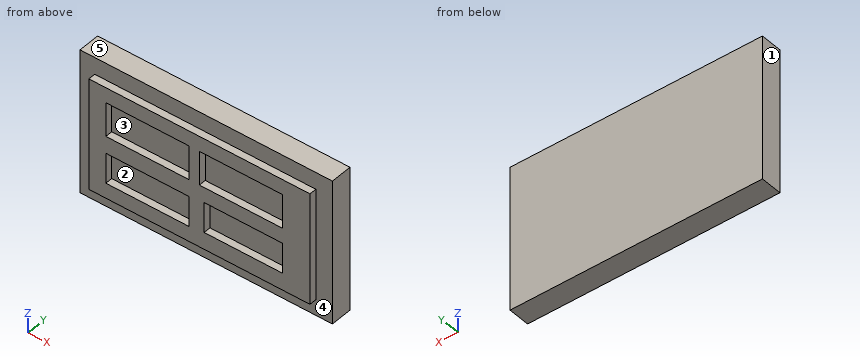
from build123d import *

# Parameters (mm, degrees)
F0_W        = 30.6613992434
F0_H        = 15.4617307708
F0_W_2      = 11.5307830274
F0_H_2      = 4.1930116713
F0_W_3      = 10.8756236732
F0_H_3      = 4.7171385959
F0_W_4      = 11.5307817468
F1_DEPTH    = 1
F0_W_5      = 35
F0_H_4      = 20
F2_DEPTH    = 2
F1_FACE_W   = 30.6613992434
F1_FACE_H   = 15.4617307708
F1_FACE_W_2 = 11.5307830274
F1_FACE_H_2 = 4.1930116713
F1_FACE_W_3 = 10.8756236732
F1_FACE_H_3 = 4.7171385959
F1_FACE_W_4 = 11.5307817468
F3_DEPTH    = 3


with BuildPart() as f1:
    # F0 (on Front) → F1 (new body)
    with BuildSketch(Plane.XZ):
        with Locations((-11.5307817468, -16.9030786492)):
            Rectangle(F0_W, F0_H)
        with Locations((-18.7375210226, -20.4409323633)):
            Rectangle(F0_W_2, F0_H_2, mode=Mode.SUBTRACT)
        with Locations((-5.4378118366, -20.1788693666)):
            Rectangle(F0_W_3, F0_H_2, mode=Mode.SUBTRACT)
        with Locations((-18.7375210226, -13.6272883974)):
            Rectangle(F0_W_2, F0_H_3, mode=Mode.SUBTRACT)
        with Locations((-5.7653908734, -13.6272883974)):
            Rectangle(F0_W_4, F0_H_3, mode=Mode.SUBTRACT)
    extrude(amount=F1_DEPTH)

    # F0 (on Front) → F2 (join)
    with BuildSketch(Plane.XZ):
        with Locations((-11.3997505978, -16.8241263426)):
            Rectangle(F0_W_5, F0_H_4)
        with Locations((-11.5307817468, -16.9030786492)):
            Rectangle(F0_W, F0_H, mode=Mode.SUBTRACT)
    extrude(amount=F2_DEPTH)

    # F0 (on Front) + F1_face (on face) → F3 (join)
    with BuildSketch(Plane.XZ):
        with Locations((-11.3997505978, -16.8241263426)):
            Rectangle(F0_W_5, F0_H_4)
        with Locations((-11.5307817468, -16.9030786492)):
            Rectangle(F0_W, F0_H, mode=Mode.SUBTRACT)
        with Locations((-5.7653908734, -13.6272883974)):
            Rectangle(F0_W_4, F0_H_3)
        with Locations((-18.7375210226, -20.4409323633)):
            Rectangle(F0_W_2, F0_H_2)
        with Locations((-5.4378118366, -20.1788693666)):
            Rectangle(F0_W_3, F0_H_2)
        with Locations((-18.7375210226, -13.6272883974)):
            Rectangle(F0_W_2, F0_H_3)
    with BuildSketch(Plane(origin=(-10.9817153045, -1, -17.0354699919), x_dir=(1, 0, 0), z_dir=(0, -1, 0))):
        with Locations((-0.5490664423, 0.1323913427)):
            Rectangle(F1_FACE_W, F1_FACE_H)
        with Locations((-7.755805718, -3.4054623714)):
            Rectangle(F1_FACE_W_2, F1_FACE_H_2, mode=Mode.SUBTRACT)
        with Locations((5.5439034679, -3.1433993748)):
            Rectangle(F1_FACE_W_3, F1_FACE_H_2, mode=Mode.SUBTRACT)
        with Locations((-7.755805718, 3.4081815945)):
            Rectangle(F1_FACE_W_2, F1_FACE_H_3, mode=Mode.SUBTRACT)
        with Locations((5.2163244311, 3.4081815945)):
            Rectangle(F1_FACE_W_4, F1_FACE_H_3, mode=Mode.SUBTRACT)
    extrude(amount=F3_DEPTH)


solid = f1.part
Design review of the part built by this model. Coordinates are the model's own, in mm. Face numbers are marked on the shaded views. A direction names the side the tool comes from. Give positions to 0.01 mm unless a question says otherwise; leave off trailing zeros. Write each loop counter-clockwise with the first axis right and the second up, starting at its lowest first coordinate (ties: lowest second). Pieces come first, ordered by that corner, then holes. Notation, with made-up numbers: M 43.25,-3 L 51.25,-3 A25 ccw 51.25,33 Z; hole C -16.5,-36.5 d4. An arc over 180 degrees is marked long. Answer as a JSON object with one key per item and string values. Group by question number.
1) We need section D-D (z = -21.5). Give the boundary of the cut face in (x, y), and give its area (3 significant figures).
2) We need section B-B (z = -10.75). Give the boundary of the cut face in (x, y).
3) Mouldability with a two-part tool opening along Z and no side actions: class the marked faces 3, 4 and 5 as released by +Z, released by -Z, zero draft, split by the parting line, or undercut.
4) For line 1 along X through (y, z) = (-3.1, -14.25); line 2 along Z through (x, y) = (-9, -3.3); line 3 along Y through (x, z) = (-17.5, -25.5), list the stretches that pass through material, from the lowest coordinate up.
5) Tool access review of the marked faces 1 and 2: name each direction out of +Z, -Z, +X, -X, +Y, -Y from which nothing blocks a thin tool from reaching the whole face with its end or side.
6) We need section A-A (y = -3.4). Give the boundary of the cut face in (x, z), and give its area (3 significant figures).
7) We need section C-C (x = -3.5). Give the boundary of the cut face in (y, z).
8) Clearance check with flat-ended pins moving along their axes: pin 1 Ø1.4 at (x, z) = (-4.5, -14) entering from -Y; pin 2 Ø0.5 at (y, z) = (-3.5, -14.5) entering from -X; pin 3 Ø0.8 at (x, y) = (-18.5, -3.5) entering from -Z. State where each tip first meets the part, or that it passes through.
Answer key:
{
 "1": {"outline": "M -28.9,-3 L -26.86,-3 L -26.86,-4 L -24.5,-4 L -24.5,-3 L -12.97,-3 L -12.97,-4 L -10.88,-4 L -10.88,-3 L 0,-3 L 0,-4 L 3.8,-4 L 3.8,-3 L 6.1,-3 L 6.1,0 L -28.9,0 Z", "area": "113 mm²"},
 "2": {"outline": "M -28.9,-3 L -26.86,-3 L -26.86,-4 L 3.8,-4 L 3.8,-3 L 6.1,-3 L 6.1,0 L -28.9,0 Z"},
 "3": {"face 3": "undercut", "face 4": "zero draft", "face 5": "released by +Z"},
 "4": {"line 1": "x = -26.86 to -24.5, -12.97 to -11.53, 0 to 3.8", "line 2": "z = -24.63 to -22.28, -18.08 to -15.99, -11.27 to -9.17", "line 3": "y = -3 to 0"},
 "5": {"face 1": "+Z, -Z, -X, +Y, -Y", "face 2": "-Y"},
 "6": {"outline": "M -26.86,-24.63 L 3.8,-24.63 L 3.8,-9.17 L -26.86,-9.17 Z; hole M -24.5,-22.54 L -12.97,-22.54 L -12.97,-18.34 L -24.5,-18.34 Z; hole M -24.5,-15.99 L -12.97,-15.99 L -12.97,-11.27 L -24.5,-11.27 Z; hole M -11.53,-15.99 L 0,-15.99 L 0,-11.27 L -11.53,-11.27 Z; hole M -10.88,-22.28 L 0,-22.28 L 0,-18.08 L -10.88,-18.08 Z", "area": "271 mm²"},
 "7": {"outline": "M -4,-24.63 L -3,-24.63 L -3,-26.82 L 0,-26.82 L 0,-6.82 L -3,-6.82 L -3,-9.17 L -4,-9.17 L -4,-11.27 L -3,-11.27 L -3,-15.99 L -4,-15.99 L -4,-18.08 L -3,-18.08 L -3,-22.28 L -4,-22.28 Z"},
 "8": {"pin 1": "stops at y = -3", "pin 2": "stops at x = -26.86", "pin 3": "stops at z = -24.63"}
}
